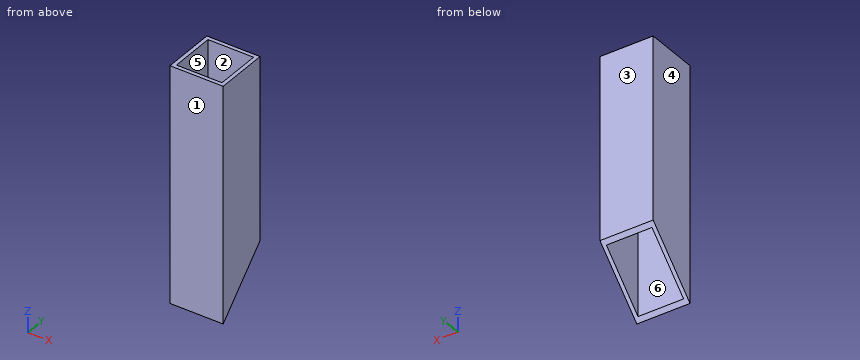
Autodesk Inventor part; units mm, degrees
ref_plane "YZ Plane" through (0, 0, 0) normal (1, 0, 0) x (0, 1, 0)
ref_plane "XZ Plane" through (0, 0, 0) normal (0, 1, 0) x (-1, 0, 0)
ref_plane "XY Plane" through (0, 0, 0) normal (0, 0, 1) x (1, 0, 0)
sketch "Sketch1" plane through (0, 0, 0) normal (0, 0, 1) x (1, 0, 0)
  line L0 (-30.5992, 26.7179) -> (13.8508, 26.7179)
  line L1 (13.8508, 26.7179) -> (13.8508, -17.7321)
  line L2 (13.8508, -17.7321) -> (-30.5992, -17.7321)
  line L3 (-30.5992, -17.7321) -> (-30.5992, 26.7179)
  dimension "d0" = 44.45
  dimension "d1" = 44.45
extrude "Extrusion1" add sketch "Sketch1" along normal blind 196.85
shell "Shell1" thickness 3.175 removed faces 2 at (-15.7825, -2.9154, 0) at (-15.7825, -2.9154, 196.85)
sketch "Sketch2" plane through (13.8508, -17.7321, 0) normal (1, 0, 0) x (0, 0, -1)
  line L0 (0, 0) -> (-196.85, 0)
  line L1 (0, 44.45) -> (0, 0)
  line L2 (0, 44.45) -> (-196.85, 44.45)
  line L3 (0, 0) -> (-44.45, 44.45)
  dimension "d5" = 45
extrude "Extrusion2" cut sketch "Sketch2" against normal through all
properties part number "FE-00001-01"
The listing builds one solid part. Answer for the finished solid, in the listing's coordinates (mm). Face numbers are marked on the shaded views. A direction names the side the tool comes from. Round coordinates to 2 decimals unless told otherwise and drop trailing zeros. Write each loop counter-clockwise with the first axis right and the second up, starting at its lowest first coordinate (ties: lowest second). Pieces come first, ordered by that corner, then holes. Notation, with made-up numbers: (59, 88) - (78, 88) arc R29 cw to (78, 126) - close; hole circle Ø4 at (32.25, 83.25). An arc over 180 degrees is marked (long way). Use a Markdown table: item, result. Add a question column.
1. The part is cut by section A-A (x = -25). Write down the section's boundary in (y, z) (3 decimals), and give its area (3 significant figures).
2. The part is cut by section B-B (y = 18.5). Write down the section's boundary in (x, z).
3. A tool of negligible diameter and unlimited length cuts with its end or side. For the marked faces 1 and 2, from which of +Z, -Z, +X, -X, +Y, -Y can it reach the whole face along a straight path? Write none if from no direction.
4. For a pull along X with two mould halves and no side action, classify the marked faces 3, 4, 5 and 6 as +X half, -X half, draft (parallel to the pull), parting line (faces both ways), or undercut.
5. The part is cut by section C-C (z = 96.5). Write down the section's boundary in (x, y), and give its area (3 significant figures).
6. Consider line 1 (Y direction, x = -4, z = 175); line 2 (X direction, y = 16.5, z = 52); line 3 (Y direction, x = -7, z = 27.5). Determine where each line is inside the solid, lowest interval first.
Reported:
| question | item | result |
|---|---|---|
| 1 | outline | (-17.732, 0) - (-14.557, 3.175) - (-14.557, 196.85) - (-17.732, 196.85) - close; (23.543, 41.275) - (26.718, 44.45) - (26.718, 196.85) - (23.543, 196.85) - close |
| 1 | area | 1,110 mm^2 |
| 2 | outline | (-30.6, 36.23) - (-27.42, 36.23) - (-27.42, 196.85) - (-30.6, 196.85) - close; (10.68, 36.23) - (13.85, 36.23) - (13.85, 196.85) - (10.68, 196.85) - close |
| 3 | face 1 | +Z, -Z, +X, -X, -Y |
| 3 | face 2 | +Z, -Z |
| 4 | face 3 | draft |
| 4 | face 4 | -X half |
| 4 | face 5 | undercut |
| 4 | face 6 | undercut |
| 5 | outline | (-30.6, -17.73) - (13.85, -17.73) - (13.85, 26.72) - (-30.6, 26.72) - close; hole (-27.42, -14.56) - (10.68, -14.56) - (10.68, 23.54) - (-27.42, 23.54) - close |
| 5 | area | 524 mm^2 |
| 6 | line 1 | -17.73 to -14.56, 23.54 to 26.72 |
| 6 | line 2 | -30.6 to -27.42, 10.68 to 13.85 |
| 6 | line 3 | -17.73 to -14.56 |
